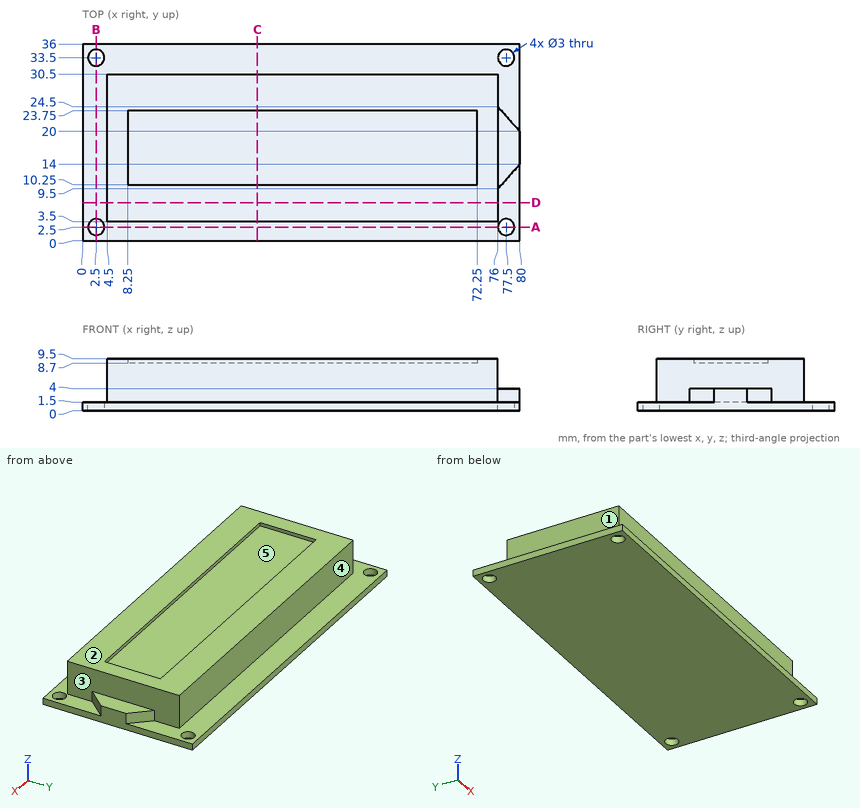
Could you check a few things on this drawing? It's one solid part, dimensions in mm from its lowest x, y, z. A direction names the side the tool comes from. Round coordinates to 2 decimals unless told otherwise and drop trailing zeros. Write each loop counter-clockwise with the first axis right and the second up, starting at its lowest first coordinate (ties: lowest second). Pieces come first, ordered by that corner, then holes. Notation, with made-up numbers: (78.5, 57) -> (116.5, 57) arc R23 ccw to (116.5, 75) -> close; hole circle Ø9 at (66, 17). An arc over 180 degrees is marked (long way). Use a Markdown table: item, result.
1. For pin 1 Ø0.9 at (x, z) = (30.5, 9) entering from +Y; pin 2 Ø4 at (y, z) = (21.5, 5.5) entering from -X; pin 3 Ø1.5 at (y, z) = (21.5, 5) entering from +X, each with a flat end and sliding along its axis, tell me the tip position at first contact or that it passes through.
Answer key:
| item | result |
|---|---|
| pin 1 | stops at y = 30.5 |
| pin 2 | stops at x = 4.5 |
| pin 3 | stops at x = 76 |
2. Which directions (+Z, -Z, +X, -X, +Y, -Y) give clear straight access to the entire face, cutting with the end or side of a thin tool? Please do the marked faces 1 and 2.
Answer key:
| item | result |
|---|---|
| face 1 | +Z, -X, +Y, -Y |
| face 2 | +Z, +X, -X, +Y, -Y |
3. If we section it at D-D (y = 7): List the corners of the cut face in (x, z) for me, then the cut area to 3 significant figures.
Answer key:
| item | result |
|---|---|
| outline | (0, 0) -> (80, 0) -> (80, 1.5) -> (76, 1.5) -> (76, 9.5) -> (4.5, 9.5) -> (4.5, 1.5) -> (0, 1.5) -> close |
| area | 692 mm^2 |
4. If we section it at B-B (x = 2.5): List the corners of the cut face in (y, z) for me, then the cut area to 3 significant figures.
Answer key:
| item | result |
|---|---|
| outline | (0, 0) -> (1, 0) -> (1, 1.5) -> (0, 1.5) -> close; (4, 0) -> (32, 0) -> (32, 1.5) -> (4, 1.5) -> close; (35, 0) -> (36, 0) -> (36, 1.5) -> (35, 1.5) -> close |
| area | 45.0 mm^2 |
5. We'd pull the mould along Y, two halves only. Please class the marked faces 3, 4 and 5: +Y half, -Y half, draft (parallel to the pull), parting line (faces both ways), or undercut.
Answer key:
| item | result |
|---|---|
| face 3 | draft |
| face 4 | +Y half |
| face 5 | undercut |
6. Please list where these lines run through material, in increasing order: probe 1 along Y at (x, z) = (77.5, 0.7); probe 2 along X at (y, z) = (19.5, 3); probe 3 along Z at (x, y) = (27, 33).
Answer key:
| item | result |
|---|---|
| probe 1 | y = 0 to 1, 4 to 32, 35 to 36 |
| probe 2 | x = 4.5 to 80 |
| probe 3 | z = 0 to 1.5 |
7. If we section it at C-C (x = 32): List the corners of the cut face in (y, z) for me, then the cut area to 3 significant figures.
Answer key:
| item | result |
|---|---|
| outline | (0, 0) -> (36, 0) -> (36, 1.5) -> (30.5, 1.5) -> (30.5, 9.5) -> (23.75, 9.5) -> (23.75, 8.7) -> (10.25, 8.7) -> (10.25, 9.5) -> (3.5, 9.5) -> (3.5, 1.5) -> (0, 1.5) -> close |
| area | 259 mm^2 |
8. If we section it at A-A (y = 2.5): List the corners of the cut face in (x, z) for me.
Answer key:
| item | result |
|---|---|
| outline | (0, 0) -> (1, 0) -> (1, 1.5) -> (0, 1.5) -> close; (4, 0) -> (76, 0) -> (76, 1.5) -> (4, 1.5) -> close; (79, 0) -> (80, 0) -> (80, 1.5) -> (79, 1.5) -> close |
